Read the model definition and answer for the solid it produces. Units are mm, in the model's axes. Coordinates: 2 decimals unless noted, no trailing zeros. Loops run counter-clockwise (first coordinate to the right, second up) from the corner with the lowest first, then second, coordinate; pieces in that order, holes last. Notation, with made-up numbers: M 37,49 L 51,49 A26 cw 51,82 Z; hole C -1.75,-10 d1. An arc over 180 degrees is marked long. Use one line per item in the form item = value. Start each with the question number.
1. The part is cut by section B-B (y = 10). Give the number of separate pieces and of enclosed holes in the cut face, plus the area to 3 significant figures.
2. Flat-ended cylindrical pins translate along their axes: pin 1 (5.5 mm diameter, centred on x = 55, y = 20, fed in from +Z); pin 2 (3.5 mm diameter, centred on x = 35, y = 0, fed in from +Z). Find the tip coordinate at first contact, or state that the pin passes through.
3. Find the intervals of material crossed by probe 1 along Y at (x, z) = (25, -3.1), in increasing order. Write a range as [from, to].
4. The part is cut by section A-A (x = 95). Give the vertices of the cut face in (y, z).
from build123d import *

# Parameters (mm, degrees)
CYLINDER102_R       = 2.1
CYLINDER102_DEPTH   = 10
ARRAY001007_X_COUNT = 10
ARRAY001007_X_PITCH = 10
ARRAY001007_Y_COUNT = 5
ARRAY001007_Y_PITCH = 10
BOX007_W            = 120
BOX007_H            = 52
BOX007_DEPTH        = 5


with BuildPart() as insert_hole_array:
    # Cylinder102 → Cylinder102 (new body)
    with BuildSketch(Plane.XY):
        Circle(CYLINDER102_R)
    extrude(amount=CYLINDER102_DEPTH)

    # Array001007 X: insert_hole array ×10


with BuildPart() as insert_hole_array_1:
    add(insert_hole_array.part)
    with Locations(*[(i * ARRAY001007_X_PITCH, 0, 0) for i in range(1, ARRAY001007_X_COUNT)]):
        add(insert_hole_array.part)

    # Array001007 Y: insert_hole array ×5


with BuildPart() as insert_hole_array_2:
    add(insert_hole_array_1.part)
    with Locations(*[(0, i * ARRAY001007_Y_PITCH, 0) for i in range(1, ARRAY001007_Y_COUNT)]):
        add(insert_hole_array_1.part)


with BuildPart() as insert_hole_array_3:
    # Array001007 placement: moved
    add(insert_hole_array_2.part.moved(Location((15, -20, -5))))


with BuildPart() as bottom_cut:
    # Box007 → Box007 (new body)
    with BuildSketch(Plane(origin=(0, -26, -5), x_dir=(1, 0, 0), z_dir=(0, 0, 1))):
        with Locations((60, 26)):
            Rectangle(BOX007_W, BOX007_H)
    extrude(amount=BOX007_DEPTH)

    # Cut005: cut insert_hole array
    add(insert_hole_array_3.part, mode=Mode.SUBTRACT)


solid = bottom_cut.part
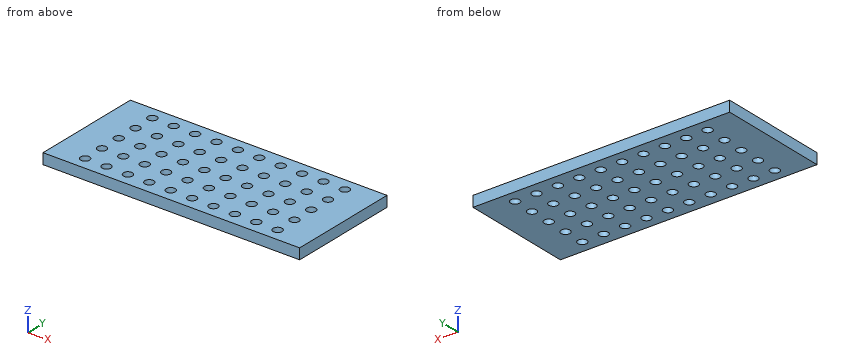
Computed values:
q1.separate_pieces = 11
q1.enclosed_holes = 0
q1.area = 390 mm²
q2.pin_1 = 0
q2.pin_2 = through
q3.probe_1 = [-26, -22.1], [-17.9, -12.1], [-7.9, -2.1], [2.1, 7.9], [12.1, 17.9], [22.1, 26]
q4.outline = M -26,-5 L -22.1,-5 L -22.1,0 L -26,0 Z; M -17.9,-5 L -12.1,-5 L -12.1,0 L -17.9,0 Z; M -7.9,-5 L -2.1,-5 L -2.1,0 L -7.9,0 Z; M 2.1,-5 L 7.9,-5 L 7.9,0 L 2.1,0 Z; M 12.1,-5 L 17.9,-5 L 17.9,0 L 12.1,0 Z; M 22.1,-5 L 26,-5 L 26,0 L 22.1,0 Z
